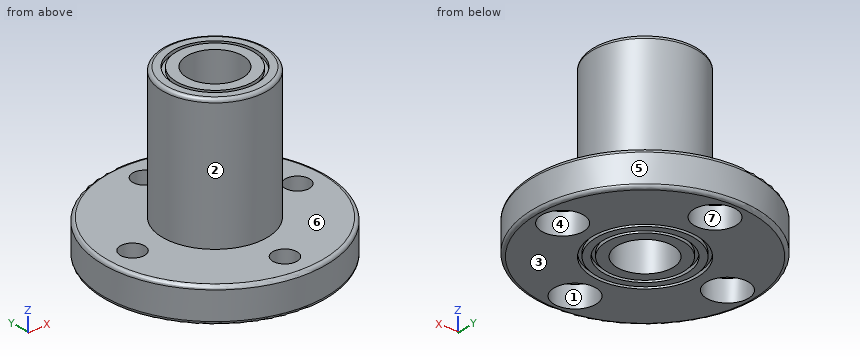
from build123d import *

# Parameters (mm, degrees)
PADR_OCIRCULAR1_COUNT = 4
FILETE1_R             = 0.5


with BuildPart() as part:
    # Esboço1 → Revolução1 (revolve)
    with BuildSketch(Plane(origin=(0, 0, 0), x_dir=(0, 0, -1), z_dir=(1, 0, 0)), mode=Mode.PRIVATE) as revolu_o1_sk:
        Polygon((0, 4), (0, 5.5), (-0.5, 5.5), (-0.5, 6), (0, 6), (0, 7), (-0.5, 7), (-0.5, 7.5), (0, 7.5), (0, 16), (-5, 16), (-5, 7.5), (-24, 7.5), (-24, 6), (-23.5, 6), (-23.5, 5.5), (-24, 5.5), (-24, 4), align=None)
    revolve(revolu_o1_sk.sketch.rotate(Axis((0, 0, 0), (0, 0, 1)), 90), axis=Axis((0, 0, 0), (0, 0, 1)))  # turned: the seam where the file's is

    # Esboço5 → Corte-Revolução1 (revolve, cut)
    with BuildSketch(Plane(origin=(0, 0, 0), x_dir=(0, 0, -1), z_dir=(1, 0, 0)), mode=Mode.PRIVATE) as corte_revolu_o1_sk:
        Polygon((0, 15), (-3.1, 15), (-3.1, 13.75), (-5, 13.75), (-5, 12), (0, 12), align=None)
    corte_revolu_o1 = revolve(corte_revolu_o1_sk.sketch.rotate(Axis((0, 12, 0), (0, 0, -1)), 180), axis=Axis((0, 12, 0), (0, 0, -1)), mode=Mode.SUBTRACT)  # turned: the seam where the file's is

    # PadrãoCircular1: Corte-Revolução1 ×4 about axis
    padr_ocircular1_axis = Axis((0, 0, 0), (0, 0, 1))
    for i in range(1, PADR_OCIRCULAR1_COUNT):
        add(corte_revolu_o1.rotate(padr_ocircular1_axis, i * 360 / PADR_OCIRCULAR1_COUNT), mode=Mode.SUBTRACT)

    # Filete1
    filete1_edges = [part.edges().sort_by_distance(p)[0] for p in [
        (7.5, 0, 24),
        (16, 0, 5),
        (16, 0, 0),
    ]]
    fillet(filete1_edges, radius=FILETE1_R)


solid = part.part
The model under review builds one solid part; all positions refer to its coordinate system, in mm. Face numbers are marked on the shaded views. A direction names the side the tool comes from. Round coordinates to 2 decimals unless told otherwise and drop trailing zeros. Loops run counter-clockwise (first coordinate to the right, second up) from the corner with the lowest first, then second, coordinate; pieces in that order, holes last. Notation, with made-up numbers: M 7,75.25 L 58,75.25 A15 cw 58,104.25 Z; hole C 54,45 d11. An arc over 180 degrees is marked long. Answer as a JSON object with one key per item and string values.
Item 1: We need section A-A, the plane z = 2. State the section outline as (x, y) points.
Check sheet entries:
{"outline": "C 0,0 d32; hole C -12,0 d6; hole C 0,0 d8; hole C 0,-12 d6; hole C 0,12 d6; hole C 12,0 d6"}
Item 2: The part is to be moulded in two halves that separate along X. For the marked faces 4, 5, 6 and 7, say which applies: +X half, -X half, draft (parallel to the pull), parting line (faces both ways), or undercut.
Check sheet entries:
{"face 4": "undercut", "face 5": "parting line", "face 6": "draft", "face 7": "undercut"}
Item 3: We need section B-B, the plane z = 5.75. State the section outline as (x, y) points.
Check sheet entries:
{"outline": "C 0,0 d15; hole C 0,0 d8"}
Item 4: For line 1 along Z through (x, y) = (2.5, 12.5); line 2 along Z through (x, y) = (3.5, 13); line 3 along X through (y, z) = (-12, 1.9), list the stretches that pass through material, from the lowest coordinate up.
Check sheet entries:
{"line 1": "3.1 to 5", "line 2": "0 to 5", "line 3": "-10.58 to -3, 3 to 10.58"}
Item 5: Clearance check with flat-ended pins moving along their axes: P1, Ø6, axis at x = -5, z = 19.5, coming from the -Y side; P2, Ø1, axis at x = 1, z = 18.5, coming from the -Y side; P3, Ø5, axis at x = -5, z = 15, coming from the -Y side. State where each tip first meets the part, or that it passes through.
Check sheet entries:
{"P1": "y = -7.23", "P2": "y = -7.48", "P3": "y = -7.07"}
Item 6: We need section C-C, the plane x = 0. State how many separate pieces and enclosed holes the cut face has, and give its area (3 significant figures).
Check sheet entries:
{"separate pieces": "4", "enclosed holes": "0", "area": "201 mm2"}
Item 7: Tool access review of the marked faces 1, 2 and 3: name each direction out of +Z, -Z, +X, -X, +Y, -Y from which nothing blocks a thin tool from reaching the whole face with its end or side.
Check sheet entries:
{"face 1": "-Z", "face 2": "+Z", "face 3": "-Z, +X, -X, +Y, -Y"}
